The listing builds one solid part. Answer for the finished solid, in the listing's coordinates (mm). A direction names the side the tool comes from. Coordinates: 2 decimals unless noted, no trailing zeros. Order: outer loops, then holes, each group sorted by start corner. A loop starts at its lowest first (then second) coordinate and runs counter-clockwise, first axis right, second up. Notation, with made-up numbers: (31.5, 0.25) -> (87.5, 0.25) arc R31 ccw to (87.5, 30.25) -> close; hole circle Ø2 at (8.5, 73.25). An arc over 180 degrees is marked (long way). One line per question, with ' | ' between items.
from build123d import *

# Parameters (mm, degrees)
SCHIZZO1_R                   = 0.5
SCHIZZO1_R_2                 = 1.25
ESTRUSIONE_ESTRUSIONE1_DEPTH = 6
RACCORDO1_R                  = 8
RACCORDO2_R                  = 40
RACCORDO3_R                  = 0.5


with BuildPart() as part:
    # Schizzo1 → Estrusione-Estrusione1 (new body)
    with BuildSketch(Plane(origin=(0, 0, 0), x_dir=(0, 0, -1), z_dir=(1, 0, 0))):
        with BuildLine():
            Line((22.6, 14.5), (2.6, 14.5))
            ThreePointArc((2.6, 14.5), (-5.9, 6), (2.6, -2.5))
            Line((2.6, -2.5), (55, -2.5))
            ThreePointArc((55, -2.5), (59.829629131, 3.794095226), (52.5, 6.830127019))
            Line((52.5, 6.830127019), (48.378061008, 4))
            Line((48.378061008, 4), (22.6, 14.5))
        make_face()
        Polygon((0, 0), (0, 12), (22.6, 12), (22.6, 0), (9, 0), (9, -1), (4, -1), (4, 0), align=None, mode=Mode.SUBTRACT)
        with Locations((-2, 6)):
            Circle(SCHIZZO1_R, mode=Mode.SUBTRACT)
        with Locations((24.6, 6)):
            Circle(SCHIZZO1_R, mode=Mode.SUBTRACT)
        with Locations((55, 2.5)):
            Circle(SCHIZZO1_R_2, mode=Mode.SUBTRACT)
    extrude(amount=ESTRUSIONE_ESTRUSIONE1_DEPTH)

    # Raccordo1
    raccordo1_edges = [part.edges().sort_by_distance(p)[0] for p in [
        (3, 4, -48.378061008),
    ]]
    fillet(raccordo1_edges, radius=RACCORDO1_R)

    # Raccordo2
    raccordo2_edges = [part.edges().sort_by_distance(p)[0] for p in [
        (3, 14.5, -22.6),
    ]]
    fillet(raccordo2_edges, radius=RACCORDO2_R)

    # Raccordo3
    raccordo3_edges = [part.edges().sort_by_distance(p)[0] for p in [
        (3, 0, -22.6),
        (3, 0, 0),
        (3, 12, 0),
        (3, 12, -22.6),
        (3, 0, -4),
        (3, -1, -4),
        (3, -1, -9),
        (3, 0, -9),
    ]]
    fillet(raccordo3_edges, radius=RACCORDO3_R - 0.0001)  # a hair under: the kernel refuses the full size


solid = part.part
Item 1: Find the intervals of material crossed by L1, parallel to Z at x = 3.05, y = 3.5; L2, parallel to Z at x = 1.1, y = 1.75; L3, parallel to Y at x = 4.7, z = -55, in increasing order.
Computed values:
L1: z = -59.9 to -55.75, -54.25 to -22.6, 0 to 5.52 | L2: z = -59.94 to -56, -54 to -22.6, 0 to 4.76 | L3: y = -2.5 to 1.25, 3.75 to 7.5
Item 2: Section B-B, the plane y = 2.5 is taken. Give the vertices of the cut face in (x, z), plus the area to 3 significant figures.
Computed values:
outline: (0, -60) -> (6, -60) -> (6, -56.25) -> (0, -56.25) -> close; (0, -53.75) -> (6, -53.75) -> (6, -22.6) -> (0, -22.6) -> close; (0, 0) -> (6, 0) -> (6, 5.15) -> (0, 5.15) -> close | area: 240 mm^2
Item 3: Section A-A, the plane x = 2.35 is taken. Count the separate pieces of the cut face and the enclosed holes in it, plus the area to 3 significant figures.
Computed values:
separate pieces: 1 | enclosed holes: 4 | area: 569 mm^2
Item 4: Section C-C, the plane z = -19.5 is taken. Give the vertices of the cut face in (x, y), plus the area to 3 significant figures.
Computed values:
outline: (0, -2.5) -> (6, -2.5) -> (6, 0) -> (0, 0) -> close; (0, 12) -> (6, 12) -> (6, 14.22) -> (0, 14.22) -> close | area: 28.3 mm^2
Item 5: For faces 1 (the face through (2.958, 8.544, -37.222)), 2 (the face through (2.958, 6.187, 5.898)), 3 (the face through (3, -1, -7)), determine the directions among +Z, -Z, +X, -X, +Y, -Y from which every point of the face is accessible in a straight line to the end or side of a thin tool.
Computed values:
face 1: +X, -X, +Y | face 2: +Z, +X, -X | face 3: +X, -X
Item 6: Determine the mould class of faces 4 (the face through (3, 0, -16)), 5 (the face through (6, 4, -27)), 6 (the face through (3.042, 13.733, -22.56)) for opening direction Y: pulls with the +Y half, pulls with the -Y half, needs draft (parallel to the pull), parting line crosses it, or undercut.
Computed values:
face 4: undercut | face 5: needs draft | face 6: pulls with the +Y half
Item 7: Each of these flat-tipped pins is pushed along its axis until it touches: pin 1 Ø1 at (x, y) = (2, 7.5) entering from -Z; pin 2 Ø2.5 at (x, z) = (4.5, -2) entering from +Y; pin 3 Ø1.5 at (x, y) = (4, 3.5) entering from -Z; pin 4 Ø1.8 at (x, y) = (3, 4.5) entering from -Z. Where does it stop, or does it pass through?
Computed values:
pin 1: stops at z = -57.18 | pin 2: stops at y = 14.5 | pin 3: stops at z = -59.99 | pin 4: stops at z = -59.88
Item 8: Section D-D, the plane z = -45 is taken. Give the vertices of the cut face in (x, y).
Computed values:
outline: (0, -2.5) -> (6, -2.5) -> (6, 5.4) -> (0, 5.4) -> close
